The listing builds one solid part. Answer for the finished solid, in the listing's coordinates (mm). A direction names the side the tool comes from. Coordinates: 2 decimals unless noted, no trailing zeros. Order: outer loops, then holes, each group sorted by start corner. A loop starts at its lowest first (then second) coordinate and runs counter-clockwise, first axis right, second up. Notation, with made-up numbers: (5, 9.25) -> (12, 9.25) arc R19 ccw to (12, 18.25) -> close; hole circle Ø5 at (-38.75, 18). An arc over 180 degrees is marked (long way). One line per question, with ' | ' between items.
from build123d import *

# Parameters (mm, degrees)
SKETCH1_W           = 30
SKETCH1_H           = 30
BOSS_EXTRUDE1_DEPTH = 5
SKETCH2_W           = 30
SKETCH2_H           = 18
BOSS_EXTRUDE2_DEPTH = 5
SKETCH3_R           = 4
CUT_EXTRUDE1_DEPTH  = 1
SKETCH4_R           = 2.5
CUT_EXTRUDE2_DEPTH  = 5
SKETCH5_R           = 2.5
CUT_EXTRUDE3_DEPTH  = 5
FILLET1_R           = 10
FILLET2_R           = 2
FILLET3_R           = 5


with BuildPart() as part:
    # Sketch1 → Boss-Extrude1 (new body)
    with BuildSketch(Plane(origin=(0, 0, 0), x_dir=(1, 0, 0), z_dir=(0, 1, 0))):
        Rectangle(SKETCH1_W, SKETCH1_H)
    extrude(amount=BOSS_EXTRUDE1_DEPTH)

    # Sketch2 → Boss-Extrude2 (add)
    with BuildSketch(Plane.ZY.offset(15)):
        with Locations((0, -4)):
            Rectangle(SKETCH2_W, SKETCH2_H)
    extrude(amount=BOSS_EXTRUDE2_DEPTH)

    # Sketch3 → Cut-Extrude1 (cut)
    with BuildSketch(Plane(origin=(-15, 0, 0), x_dir=(0, 0, -1), z_dir=(1, 0, 0))):
        with Locations((-8, -5.5)):
            Circle(SKETCH3_R)
        with Locations((8, -5.5)):
            Circle(SKETCH3_R)
    extrude(amount=-CUT_EXTRUDE1_DEPTH, mode=Mode.SUBTRACT)

    # Sketch4 → Cut-Extrude2 (cut)
    with BuildSketch(Plane(origin=(-16, 0, 0), x_dir=(0, 0, -1), z_dir=(1, 0, 0))):
        with Locations((-8, -5.5)):
            Circle(SKETCH4_R)
        with Locations((8, -5.5)):
            Circle(SKETCH4_R)
    extrude(amount=-CUT_EXTRUDE2_DEPTH, mode=Mode.SUBTRACT)

    # Sketch5 → Cut-Extrude3 (cut)
    with BuildSketch(Plane(origin=(0, 5, 0), x_dir=(1, 0, 0), z_dir=(0, 1, 0))):
        with Locations((-1.75, 0)):
            Circle(SKETCH5_R)
    extrude(amount=-CUT_EXTRUDE3_DEPTH, mode=Mode.SUBTRACT)

    # Fillet1
    fillet1_edges = [part.edges().sort_by_distance(p)[0] for p in [
        (15, 2.5, -15),
        (15, 2.5, 15),
    ]]
    fillet(fillet1_edges, radius=FILLET1_R)

    # Fillet2
    fillet2_edges = [part.edges().sort_by_distance(p)[0] for p in [
        (-15, 0, 0),
    ]]
    fillet(fillet2_edges, radius=FILLET2_R)

    # Fillet3
    fillet3_edges = [part.edges().sort_by_distance(p)[0] for p in [
        (-17.5, -13, -15),
        (-17.5, -13, 15),
    ]]
    fillet(fillet3_edges, radius=FILLET3_R)


solid = part.part
Item 1: For faces 1 (the face through (-16, -5, -11)), 2 (the face through (15, 2, 0)), 3 (the face through (-15, -9, 0)), determine the directions among +Z, -Z, +X, -X, +Y, -Y from which every point of the face is accessible in a straight line to the end or side of a thin tool.
Computed values:
face 1: +X | face 2: +Z, -Z, +X, +Y, -Y | face 3: +Z, -Z, +X, -Y
Item 2: Each of these flat-tipped pins is pushed along its axis until it touches: pin 1 Ø4.5 at (y, z) = (-5.5, 8) entering from -X; pin 2 Ø8.5 at (x, z) = (6, -3) entering from -Y; pin 3 Ø7 at (y, z) = (-5.5, 8) entering from +X; pin 4 Ø9 at (y, z) = (-6.5, -10) entering from +X. Where does it stop, or does it pass through?
Computed values:
pin 1: passes through | pin 2: stops at y = 0 | pin 3: stops at x = -16 | pin 4: stops at x = -15
Item 3: Section D-D, the plane y = 1.25 is taken. Give the vertices of the cut face in (x, z), plus the area to 3 significant figures.
Computed values:
outline: (-20, -15) -> (5, -15) arc R10 ccw to (15, -5) -> (15, 5) arc R10 ccw to (5, 15) -> (-20, 15) -> close; hole circle Ø5 at (-1.75, 0) | area: 987 mm^2
Item 4: Find the intervals of material crossed by L1, parallel to Z at x = -15.7, y = -5.5; L2, parallel to X at y = -10.5, z = 0.5; L3, parallel to Y at x = -17.05, z = 8, in increasing order.
Computed values:
L1: z = -15 to -12, -4 to 4, 12 to 15 | L2: x = -20 to -15 | L3: y = -13 to -8, -3 to 5
Item 5: Determine the mould class of faces 4 (the face through (-17, -13, 0)), 5 (the face through (12.15, 2.54, 11.99)), 6 (the face through (-4.248, 2.535, -0.11)) for opening direction X: pulls with the +X half, pulls with the -X half, needs draft (parallel to the pull), parting line crosses it, or undercut.
Computed values:
face 4: needs draft | face 5: pulls with the +X half | face 6: undercut
Item 6: Section B-B, the plane y = -5.5 is taken. Give the vertices of the cut face in (x, z), plus the area to 3 significant figures.
Computed values:
outline: (-20, -15) -> (-15, -15) -> (-15, -12) -> (-16, -12) -> (-16, -10.5) -> (-20, -10.5) -> close; (-20, -5.5) -> (-16, -5.5) -> (-16, -4) -> (-15, -4) -> (-15, 4) -> (-16, 4) -> (-16, 5.5) -> (-20, 5.5) -> close; (-20, 10.5) -> (-16, 10.5) -> (-16, 12) -> (-15, 12) -> (-15, 15) -> (-20, 15) -> close | area: 94.0 mm^2
Item 7: Section A-A, the plane z = 0 is taken. Give the vertices of the cut face in (x, y).
Computed values:
outline: (-20, -13) -> (-15, -13) -> (-15, -2) arc R2 cw to (-13, 0) -> (-4.25, 0) -> (-4.25, 5) -> (-20, 5) -> close; (0.75, 0) -> (15, 0) -> (15, 5) -> (0.75, 5) -> close
Item 8: Section C-C, the plane x = -1.75 is taken. Give the vertices of the cut face in (y, z).
Computed values:
outline: (0, -15) -> (5, -15) -> (5, -2.5) -> (0, -2.5) -> close; (0, 2.5) -> (5, 2.5) -> (5, 15) -> (0, 15) -> close
